Read the model definition and answer for the solid it produces. Units are mm, in the model's axes. A direction names the side the tool comes from. Give positions to 0.01 mm unless a question says otherwise; leave off trailing zeros. Loops run counter-clockwise (first coordinate to the right, second up) from the corner with the lowest first, then second, coordinate; pieces in that order, holes last. Notation, with made-up numbers: (-6.75, 73) - (24.25, 73) arc R22 ccw to (24.25, 109) - close; hole circle Ø3 at (-31.5, 70.5). An arc over 180 degrees is marked (long way). Write item = value, one per line.
```python
from build123d import *

# Parameters (mm, degrees)
SKETCH1_R           = 1.397
BOSS_EXTRUDE1_DEPTH = 31.75
SKETCH2_R           = 2.286
BOSS_EXTRUDE2_DEPTH = 2.54
CUT_EXTRUDE1_DEPTH  = 1.905


with BuildPart() as part:
    # Sketch1 → Boss-Extrude1 (new body)
    with BuildSketch(Plane.XY):
        Circle(SKETCH1_R)
    extrude(amount=BOSS_EXTRUDE1_DEPTH)

    # Sketch2 → Boss-Extrude2 (add)
    with BuildSketch(Plane.XY.offset(31.75)):
        Circle(SKETCH2_R)
    extrude(amount=BOSS_EXTRUDE2_DEPTH)

    # Sketch4 → Cut-Extrude1 (cut)
    with BuildSketch(Plane.XY.offset(34.29)):
        Polygon((1.566413347, -0.889919011), (1.553899145, 0.911594246), (-0.012514203, 1.801513257), (-1.566413347, 0.889919011), (-1.553899145, -0.911594246), (0.012514203, -1.801513257), align=None)
    extrude(amount=-CUT_EXTRUDE1_DEPTH, mode=Mode.SUBTRACT)


solid = part.part
```
1) Find the intervals of material crossed by probe 1 along Z at (x, y) = (0.25, -1) (3 decimals); probe 2 along Z at (x, y) = (-0.4, -1.7); probe 3 along Y at (x, z) = (0.5, 7), in increasing order.
Output:
probe_1 = 0 to 32.385
probe_2 = 31.75 to 34.29
probe_3 = -1.3 to 1.3
2) This flat-tipped pin is pushed along its axis until it touches: P1, Ø0.9, axis at x = 0, y = -0.5, coming from the +Z side (3 decimals). Where does it stop, or does it pass through?
Output:
P1 = 32.385
3) A tool of negligible diameter and unlimited length cuts with its end or side. For faces 4 (the face through (-1.11, -0.85, 15.65)), 5 (the face through (0.78, 1.35, 33.35)), 6 (the face through (0, 2, 34.29)), from which of +Z, -Z, +X, -X, +Y, -Y can it reach the whole face along a straight path? Write none if from no direction.
Output:
face_4 = -Z
face_5 = +Z
face_6 = +Z, +X, -X, +Y, -Y
4) A cutting plane is placed at B-B on z = 16. Determine the outline of the cut face in (x, y), then the cut area to 3 significant figures.
Output:
outline = circle Ø2.79 at (0, 0)
area = 6.13 mm²
5) The mould has two halves that part along X. Classify faces 1 (the face through (-0.78, -1.35, 33.35)), 2 (the face through (0.5, -1.5, 31.75)), 3 (the face through (-0.5, -2.23, 33)): pulls with the +X half, pulls with the -X half, needs draft (parallel to the pull), parting line crosses it, or undercut.
Output:
face_1 = undercut
face_2 = needs draft
face_3 = parting line crosses it
6) A cutting plane is placed at C-C on x = -0.9. Determine the outline of the cut face in (y, z) (3 decimals).
Output:
outline = (-2.101, 31.75) - (-1.068, 31.75) - (-1.068, 0) - (1.068, 0) - (1.068, 31.75) - (2.101, 31.75) - (2.101, 34.29) - (1.281, 34.29) - (1.281, 32.385) - (-1.283, 32.385) - (-1.283, 34.29) - (-2.101, 34.29) - close
